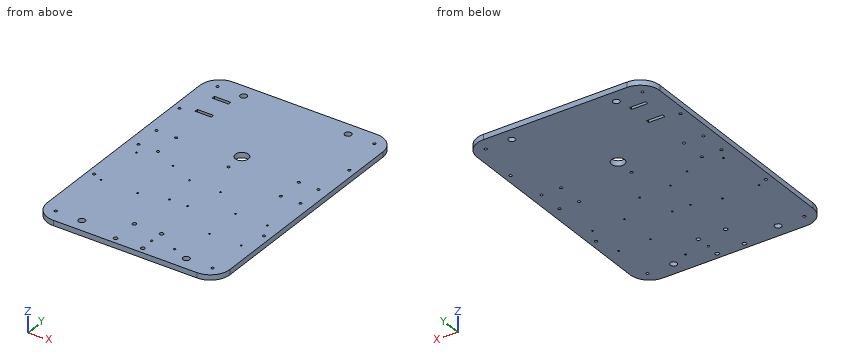
```python
from build123d import *

# Parameters (mm, degrees)
CYLINDER006_R            = 2.1
CYLINDER006_DEPTH        = 60
ARRAY004_X_COUNT         = 2
ARRAY004_X_PITCH         = 30
ARRAY004_Y_COUNT         = 2
ARRAY004_Y_PITCH         = 40
ARRAY005_COUNT           = 2
CYLINDER003_R            = 5.1
CYLINDER003_DEPTH        = 70
ARRAY002_X_COUNT         = 2
ARRAY002_X_PITCH         = 160
SKETCH001_R              = 1.25
PAD001_DEPTH             = 50
CLONE_PLACEMENT_ANGLE    = -90
CYLINDER008_R            = 1.25
CYLINDER008_DEPTH        = 60
ARRAY007_X_COUNT         = 2
ARRAY007_X_PITCH         = 55.88
ARRAY007_Y_COUNT         = 2
ARRAY007_Y_PITCH         = 78.74
SKETCH002_R              = 1.2
PAD003_DEPTH             = 50
CLONE001_PLACEMENT_ANGLE = -90
BOX013_W                 = 25
BOX013_H                 = 5
BOX013_DEPTH             = 50
ARRAY035_Y_COUNT         = 2
ARRAY035_Y_PITCH         = 38
CYLINDER034_R            = 5.1
CYLINDER034_DEPTH        = 70
ARRAY033_X_COUNT         = 2
ARRAY033_X_PITCH         = 160
CYLINDER035_R            = 2.1
CYLINDER035_DEPTH        = 120
ARRAY036_X_COUNT         = 2
ARRAY036_X_PITCH         = 240
ARRAY036_Y_COUNT         = 2
ARRAY036_Y_PITCH         = 360
CYLINDER036_R            = 2.1
CYLINDER036_DEPTH        = 110
ARRAY037_X_COUNT         = 2
ARRAY037_X_PITCH         = 260
ARRAY037_Y_COUNT         = 2
ARRAY037_Y_PITCH         = 190
CYLINDER037_R            = 2.1
CYLINDER037_DEPTH        = 120
CYLINDER005_R            = 3
CYLINDER005_DEPTH        = 50
ARRAY003_COUNT           = 4
CYLINDER039_R            = 1.6
CYLINDER039_DEPTH        = 50
ARRAY038_X_COUNT         = 2
ARRAY038_X_PITCH         = 35
CYLINDER007_R            = 10
CYLINDER007_DEPTH        = 50
BOX002_W                 = 280
BOX002_H                 = 400
BOX002_DEPTH             = 8
FILLET_R                 = 30


with BuildPart() as obj1:
    # Cylinder006 → Cylinder006 (new body)
    with BuildSketch(Plane(origin=(16, -20, 0), x_dir=(1, 0, 0), z_dir=(0, 0, 1))):
        Circle(CYLINDER006_R)
    extrude(amount=CYLINDER006_DEPTH)

    # Array004 X: obj1_2


with BuildPart() as obj1_1:
    add(obj1.part)
    with Locations(*[(i * ARRAY004_X_PITCH, 0, 0) for i in range(1, ARRAY004_X_COUNT)]):
        add(obj1.part)

    # Array004 Y: obj1_2


with BuildPart() as obj1_2:
    add(obj1_1.part)
    with Locations(*[(0, i * ARRAY004_Y_PITCH, 0) for i in range(1, ARRAY004_Y_COUNT)]):
        add(obj1_1.part)

    # Array005: obj1_2 about axis
    array005_axis = Axis((140, 0, 0), (0, 0, 1))


with BuildPart() as obj1_3:
    add(obj1_2.part)
    for i in range(1, ARRAY005_COUNT):
        add(obj1_2.part.rotate(array005_axis, i * 360 / ARRAY005_COUNT))


with BuildPart() as obj2:
    # Cylinder003 → Cylinder003 (new body)
    with BuildSketch(Plane(origin=(60, -210, -13), x_dir=(1, 0, 0), z_dir=(0, 0, 1))):
        Circle(CYLINDER003_R)
    extrude(amount=CYLINDER003_DEPTH)

    # Array002 X: obj2_ ×2


with BuildPart() as obj2_1:
    add(obj2.part)
    with Locations(*[(i * ARRAY002_X_PITCH, 0, 0) for i in range(1, ARRAY002_X_COUNT)]):
        add(obj2.part)


with BuildPart() as clone_of_arduino_uno_holes:
    # Sketch001 → Pad001 (new body)
    with BuildSketch(Plane.XY):
        with Locations((14, 2.5)):
            Circle(SKETCH001_R)
        with Locations((15.3, 50.7)):
            Circle(SKETCH001_R)
        with Locations((66.1, 35.5)):
            Circle(SKETCH001_R)
        with Locations((66.1, 7.6)):
            Circle(SKETCH001_R)
    extrude(amount=PAD001_DEPTH)


with BuildPart() as clone_of_arduino_uno_holes_1:
    # Clone placement: moved
    add(clone_of_arduino_uno_holes.part.moved(Location((115, -40, 0))).rotate(Axis((115, -40, 0), (0, 0, 1)), CLONE_PLACEMENT_ANGLE))


with BuildPart() as array007:
    # Cylinder008 → Cylinder008 (new body)
    with BuildSketch(Plane(origin=(25.06, -37.63, 0), x_dir=(1, 0, 0), z_dir=(0, 0, 1))):
        Circle(CYLINDER008_R)
    extrude(amount=CYLINDER008_DEPTH)

    # Array007 X: Array007 ×2


with BuildPart() as array007_1:
    add(array007.part)
    with Locations(*[(i * ARRAY007_X_PITCH, 0, 0) for i in range(1, ARRAY007_X_COUNT)]):
        add(array007.part)

    # Array007 Y: Array007 ×2


with BuildPart() as array007_2:
    add(array007_1.part)
    with Locations(*[(0, -i * ARRAY007_Y_PITCH, 0) for i in range(1, ARRAY007_Y_COUNT)]):
        add(array007_1.part)


with BuildPart() as mount_electronics:
    # Sketch002 → Pad003 (new body)
    with BuildSketch(Plane.XY.offset(-4)):
        with Locations((-39, 24.5)):
            Circle(SKETCH002_R)
        with Locations((19, 24.5)):
            Circle(SKETCH002_R)
        with Locations((-39, -24.5)):
            Circle(SKETCH002_R)
        with Locations((19, -24.5)):
            Circle(SKETCH002_R)
    extrude(amount=PAD003_DEPTH)


with BuildPart() as mount_electronics_1:
    # Clone001 placement: moved
    add(mount_electronics.part.moved(Location((235, -126, 0))).rotate(Axis((235, -126, 0), (0, 0, 1)), CLONE001_PLACEMENT_ANGLE))

    # Fusion002: union Clone of arduino_uno_holes_, Array007
    add(clone_of_arduino_uno_holes_1.part)
    add(array007_2.part)


with BuildPart() as array035:
    # Box013 → Box013 (new body)
    with BuildSketch(Plane(origin=(30, 123.5, 0), x_dir=(1, 0, 0), z_dir=(0, 0, 1))):
        with Locations((12.5, 2.5)):
            Rectangle(BOX013_W, BOX013_H)
    extrude(amount=BOX013_DEPTH)

    # Array035 Y: Array035 ×2


with BuildPart() as array035_1:
    add(array035.part)
    with Locations(*[(0, -i * ARRAY035_Y_PITCH, 0) for i in range(1, ARRAY035_Y_COUNT)]):
        add(array035.part)


with BuildPart() as obj3:
    # Cylinder034 → Cylinder034 (new body)
    with BuildSketch(Plane(origin=(60, 150, -13), x_dir=(1, 0, 0), z_dir=(0, 0, 1))):
        Circle(CYLINDER034_R)
    extrude(amount=CYLINDER034_DEPTH)

    # Array033 X: obj3 ×2


with BuildPart() as obj3_1:
    add(obj3.part)
    with Locations(*[(i * ARRAY033_X_PITCH, 0, 0) for i in range(1, ARRAY033_X_COUNT)]):
        add(obj3.part)


with BuildPart() as array036:
    # Cylinder035 → Cylinder035 (new body)
    with BuildSketch(Plane(origin=(20, -210, 0), x_dir=(1, 0, 0), z_dir=(0, 0, 1))):
        Circle(CYLINDER035_R)
    extrude(amount=CYLINDER035_DEPTH)

    # Array036 X: Array036 ×2


with BuildPart() as array036_1:
    add(array036.part)
    with Locations(*[(i * ARRAY036_X_PITCH, 0, 0) for i in range(1, ARRAY036_X_COUNT)]):
        add(array036.part)

    # Array036 Y: Array036 ×2


with BuildPart() as array036_2:
    add(array036_1.part)
    with Locations(*[(0, i * ARRAY036_Y_PITCH, 0) for i in range(1, ARRAY036_Y_COUNT)]):
        add(array036_1.part)


with BuildPart() as array037:
    # Cylinder036 → Cylinder036 (new body)
    with BuildSketch(Plane(origin=(10, -110, 0), x_dir=(1, 0, 0), z_dir=(0, 0, 1))):
        Circle(CYLINDER036_R)
    extrude(amount=CYLINDER036_DEPTH)

    # Array037 X: Array037 ×2


with BuildPart() as array037_1:
    add(array037.part)
    with Locations(*[(i * ARRAY037_X_PITCH, 0, 0) for i in range(1, ARRAY037_X_COUNT)]):
        add(array037.part)

    # Array037 Y: Array037 ×2


with BuildPart() as array037_2:
    add(array037_1.part)
    with Locations(*[(0, i * ARRAY037_Y_PITCH, 0) for i in range(1, ARRAY037_Y_COUNT)]):
        add(array037_1.part)


with BuildPart() as central_entretoise_m4:
    # Cylinder037 → Cylinder037 (new body)
    with BuildSketch(Plane(origin=(140, 0, 0), x_dir=(1, 0, 0), z_dir=(0, 0, 1))):
        Circle(CYLINDER037_R)
    extrude(amount=CYLINDER037_DEPTH)


with BuildPart() as array003:
    # Cylinder005 → Cylinder005 (new body)
    with BuildSketch(Plane(origin=(160.85965, -179.14035, 0), x_dir=(1, 0, 0), z_dir=(0, 0, 1))):
        Circle(CYLINDER005_R)
    extrude(amount=CYLINDER005_DEPTH)

    # Array003: Array003 ×4 about axis
    array003_axis = Axis((140, -200, 0), (0, 0, 1))


with BuildPart() as array003_1:
    add(array003.part)
    for i in range(1, ARRAY003_COUNT):
        add(array003.part.rotate(array003_axis, i * 360 / ARRAY003_COUNT))


with BuildPart() as mount_cam_pi:
    # Cylinder039 → Cylinder039 (new body)
    with BuildSketch(Plane(origin=(160, -200, 0), x_dir=(1, 0, 0), z_dir=(0, 0, 1))):
        Circle(CYLINDER039_R)
    extrude(amount=CYLINDER039_DEPTH)

    # Array038 X: mount_cam_pi_ ×2


with BuildPart() as mount_cam_pi_1:
    add(mount_cam_pi.part)
    with Locations(*[(i * ARRAY038_X_PITCH, 0, 0) for i in range(1, ARRAY038_X_COUNT)]):
        add(mount_cam_pi.part)


with BuildPart() as fusion001:
    # Cylinder007 → Cylinder007 (new body)
    with BuildSketch(Plane(origin=(140, 30, 0), x_dir=(1, 0, 0), z_dir=(0, 0, 1))):
        Circle(CYLINDER007_R)
    extrude(amount=CYLINDER007_DEPTH)

    # Fusion001: union obj1_, obj2_, mount_electronics_, Array035, obj3, Array036, Array037, central_entretoise_m4_, Array003, mount_cam_pi_
    add(obj1_3.part)
    add(obj2_1.part)
    add(mount_electronics_1.part)
    add(array035_1.part)
    add(obj3_1.part)
    add(array036_2.part)
    add(array037_2.part)
    add(central_entretoise_m4.part)
    add(array003_1.part)
    add(mount_cam_pi_1.part)


with BuildPart() as cut:
    # Box002 → Box002 (new body)
    with BuildSketch(Plane(origin=(0, -230, 29), x_dir=(1, 0, 0), z_dir=(0, 0, 1))):
        with Locations((140, 200)):
            Rectangle(BOX002_W, BOX002_H)
    extrude(amount=BOX002_DEPTH)

    # Fillet
    fillet_edges = [cut.edges().sort_by_distance(p)[0] for p in [
        (0, -230, 33),
        (0, 170, 33),
        (280, -230, 33),
        (280, 170, 33),
    ]]
    fillet(fillet_edges, radius=FILLET_R)

    # Cut: cut Fusion001
    add(fusion001.part, mode=Mode.SUBTRACT)


solid = cut.part
```
Geometry: final body of the model. Coordinates: model frame, mm. Coordinates: 2 decimals unless noted, no trailing zeros. Loops run counter-clockwise (first coordinate to the right, second up) from the corner with the lowest first, then second, coordinate; pieces in that order, holes last. Notation, with made-up numbers: M 20,-16 L 28,-16 A19 ccw 28,1 Z; hole C -12,-31 d2. An arc over 180 degrees is marked long. Put each result on its own line as item: value.
(1) Cut plane B-B on x = 220. Return the cut outline in (y, z), then the cut area to 3 significant figures.
Answer sheet:
outline: M -230,29 L -215.1,29 L -215.1,37 L -230,37 Z; M -204.9,29 L 144.9,29 L 144.9,37 L -204.9,37 Z; M 155.1,29 L 170,29 L 170,37 L 155.1,37 Z
area: 3,040 mm^2
(2) Material intervals for probe 1 along Y at (x, z) = (80.94, 31); probe 2 along Y at (x, z) = (46, 33.5); probe 3 along Y at (x, z) = (140, 31.75), sorted ascending.
Answer sheet:
probe 1: y = -230 to -117.62, -115.12 to -38.88, -36.38 to 170
probe 2: y = -230 to -22.1, -17.9 to 17.9, 22.1 to 85.5, 90.5 to 123.5, 128.5 to 170
probe 3: y = -230 to -2.1, 2.1 to 20, 40 to 170
(3) Cut plane C-C on z = 30.25. State how many separate pieces and enclosed holes the cut face has, then the cut area to 3 significant figures.
Answer sheet:
separate pieces: 1
enclosed holes: 42
area: 110,000 mm^2
(4) Cut plane A-A on x = 38. Return the cut outline in (y, z), then the cut area to 3 significant figures.
Answer sheet:
outline: M -230,29 L 85.5,29 L 85.5,37 L -230,37 Z; M 90.5,29 L 123.5,29 L 123.5,37 L 90.5,37 Z; M 128.5,29 L 170,29 L 170,37 L 128.5,37 Z
area: 3,120 mm^2
(5) First-contact query: pin 1 (3 mm diameter, centred on x = 259.5, y = -145, fed in from +Z). Flat tip, straight axial feed; report the tip coordinate or a pass-through.
Answer sheet:
pin 1: stops at z = 37
